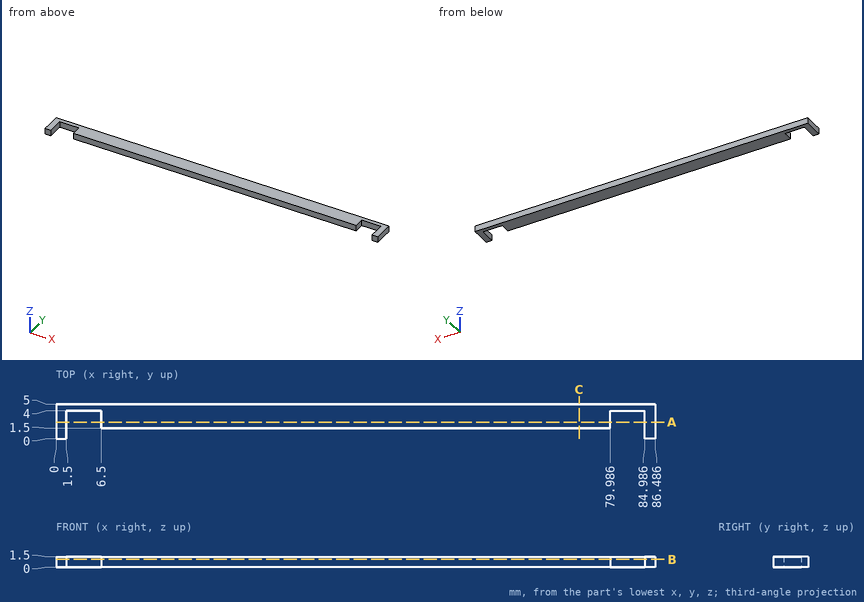
Design review of the part shown in the three views and the two pictorial views. Dimensions are in mm from the part's minimum x, y and z. Round coordinates to 2 decimals unless told otherwise and drop trailing zeros. Write each loop counter-clockwise with the first axis right and the second up, starting at its lowest first coordinate (ties: lowest second). Pieces come first, ordered by that corner, then holes.
Item 1: Clearance check with flat-ended pins moving along their axes: pin 1 Ø0.8 at (y, z) = (3, 0.5) entering from -X; pin 2 Ø0.8 at (x, z) = (4, 0.5) entering from -Y. State where each tip first meets the part, or that it passes through.
Item 2: We need section A-A on y = 2.4. Write out the cut boundary in (x, z), and give its area (3 significant figures).
Item 3: We need section C-C on x = 75.5. Write out the cut boundary in (y, z), and give its area (3 significant figures).
Item 4: For probe 1 along X at (y, z) = (3.4, 0.55); probe 2 along X at (y, z) = (0.4, 0.6); probe 3 along Y at (x, z) = (76, 1.45), list the stretches that pass through material, from the lowest coordinate up.
Item 5: We need section B-B on z = 1.1. Write out the cut boundary in (x, y).
Returned:
1. pin 1: stops at x = 0
1. pin 2: stops at y = 4
2. outline: (0, 0) - (1.5, 0) - (1.5, 1.5) - (0, 1.5) - close; (6.5, 0) - (79.99, 0) - (79.99, 1.5) - (6.5, 1.5) - close; (84.99, 0) - (86.49, 0) - (86.49, 1.5) - (84.99, 1.5) - close
2. area: 115 mm2
3. outline: (1.5, 0) - (5, 0) - (5, 1.5) - (1.5, 1.5) - close
3. area: 5.25 mm2
4. probe 1: x = 0 to 1.5, 6.5 to 79.99, 84.99 to 86.49
4. probe 2: x = 0 to 1.5, 84.99 to 86.49
4. probe 3: y = 1.5 to 5
5. outline: (0, 0) - (1.5, 0) - (1.5, 4) - (6.5, 4) - (6.5, 1.5) - (79.99, 1.5) - (79.99, 4) - (84.99, 4) - (84.99, 0) - (86.49, 0) - (86.49, 5) - (0, 5) - close
